Could you check a few things on this model? Use its own coordinates, in mm. A direction names the side the tool comes from. Give positions to 0.01 mm unless a question says otherwise; leave off trailing zeros. Loops run counter-clockwise (first coordinate to the right, second up) from the corner with the lowest first, then second, coordinate; pieces in that order, holes last. Notation, with made-up numbers: (17, 59.25) -> (76, 59.25) arc R25 cw to (76, 86.25) -> close; hole circle Ø9 at (-9, -13). An arc over 180 degrees is marked (long way). Put each result on its own line as item: value.
```python
from build123d import *

# Parameters (mm, degrees)
F0_W     = 609.6
F0_H     = 914.4
F1_DEPTH = 609.6
F2_DEPTH = 25.4
F3_T     = -3.302
F4_W     = 533.4
F4_H     = 838.2
F5_DEPTH = 584.2


with BuildPart() as f1:
    # F0 (on Front) → F1 (new body)
    with BuildSketch(Plane.XZ):
        with Locations((-127.1454390585, -4.6617306446)):
            Rectangle(F0_W, F0_H)
    extrude(amount=F1_DEPTH)

    # F2 (add): a face of the model
    f2_faces = [f1.faces().sort_by_distance(p)[0] for p in [
        (-127.1454390585, -609.6, -4.6617306446),
    ]]
    extrude(f2_faces, amount=F2_DEPTH)

    # F3 (hollow: no face is removed)
    offset(amount=F3_T, mode=Mode.SUBTRACT)

    # F4 (on face) → F5 (cut)
    with BuildSketch(Plane.XZ.offset(635)):
        with Locations((-127.1454390585, -4.6617306446)):
            Rectangle(F4_W, F4_H)
    extrude(amount=-F5_DEPTH, mode=Mode.SUBTRACT)


solid = f1.part
```
1. Thinking about a two-plate mould opening in Z: for faces 3 (the face through (-400, -635, 31)), 4 (the face through (-131, -313, 452.538)), 5 (the face through (-131, -313, -458.56)), which applies, pulls with the +Z half, pulls with the -Z half, needs draft (parallel to the pull), parting line crosses it, or undercut?
Recorded:
face 3: needs draft
face 4: pulls with the +Z half
face 5: undercut
2. If we section it at A-A (y = -496): List the corners of the cut face in (x, z) for me.
Recorded:
outline: (-431.95, -461.86) -> (177.65, -461.86) -> (177.65, 452.54) -> (-431.95, 452.54) -> close; hole (-428.64, -458.56) -> (174.35, -458.56) -> (174.35, 449.24) -> (-428.64, 449.24) -> close
3. For faces 1 (the face through (177.655, -313, -11)), 2 (the face through (-131, -313, 449.236)), which set-ups out of +Z, -Z, +X, -X, +Y, -Y let a thin tool reach every point of the face, with its end or its side?
Recorded:
face 1: +Z, -Z, +X, +Y, -Y
face 2: none
4. If we section it at C-C (z = 143): List the corners of the cut face in (x, y) for me, then the cut area to 3 significant figures.
Recorded:
outline: (-431.95, -635) -> (-393.85, -635) -> (-393.85, -631.7) -> (-428.64, -631.7) -> (-428.64, -3.3) -> (174.35, -3.3) -> (174.35, -631.7) -> (139.55, -631.7) -> (139.55, -635) -> (177.65, -635) -> (177.65, 0) -> (-431.95, 0) -> close
area: 6,410 mm^2
5. I'm going to push a flat-ended pin straight in: pin 1 (12 mm diameter, centred on x = -341, z = -161, fed in from -Y). Where does the tip first touch, or does it pass through?
Recorded:
pin 1: stops at y = -3.3
6. I need wall thicknesses on line 1 (Z direction, x = -156.5, y = -109.5); line 2 (X direction, y = -397.5, z = -246); line 3 (Y direction, x = -26, z = -27.5). Which ranges of each line are inside material? Lowest first, please.
Recorded:
line 1: z = -461.86 to -458.56, 449.24 to 452.54
line 2: x = -431.95 to -428.64, 174.35 to 177.65
line 3: y = -3.3 to 0
7. If we section it at B-B (x = 111): List the corners of the cut face in (y, z) for me.
Recorded:
outline: (-635, -461.86) -> (0, -461.86) -> (0, 452.54) -> (-635, 452.54) -> (-635, 414.44) -> (-631.7, 414.44) -> (-631.7, 449.24) -> (-3.3, 449.24) -> (-3.3, -458.56) -> (-631.7, -458.56) -> (-631.7, -423.76) -> (-635, -423.76) -> close
